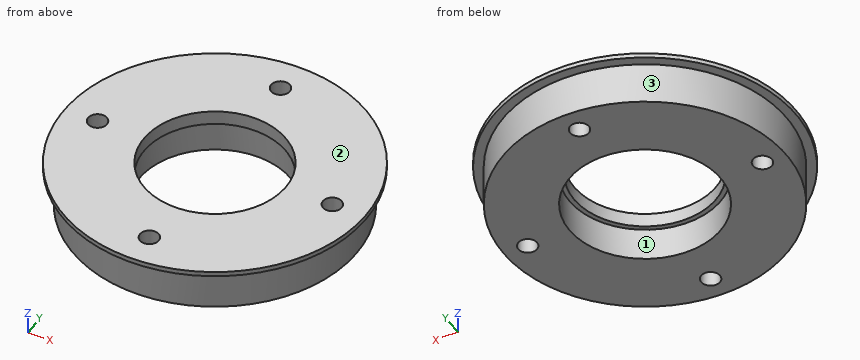
```python
from build123d import *

# Parameters (mm, degrees)
SKETCH1_R           = 29.9974
SKETCH1_R_2         = 16
BOSS_EXTRUDE1_DEPTH = 7
SKETCH2_R           = 2
CUT_EXTRUDE1_DEPTH  = 10
SKETCH3_R           = 16
SKETCH3_R_2         = 15
BOSS_EXTRUDE2_DEPTH = 1
BOSS_EXTRUDE3_START = 3
SKETCH1_3_R         = 29.9974
SKETCH1_3_R_2       = 16
BOSS_EXTRUDE3_DEPTH = 3
BOSS_EXTRUDE4_START = 2
SKETCH3_2_R         = 16
SKETCH3_2_R_2       = 15
BOSS_EXTRUDE4_DEPTH = 2
SKETCH4_R           = 31.9974
SKETCH4_R_2         = 29.9974
BOSS_EXTRUDE5_DEPTH = 1
CUT_EXTRUDE3_START  = -1
SKETCH5_R           = 16
SKETCH5_R_2         = 15
CUT_EXTRUDE3_DEPTH  = 1
SKETCH6_R           = 3
SKETCH6_R_2         = 2
BOSS_EXTRUDE6_DEPTH = 3
CHAMFER1_SIZE       = 3
CUT_EXTRUDE4_START  = -10
SKETCH7_R           = 2
CUT_EXTRUDE4_DEPTH  = 10
BOSS_EXTRUDE7_START = 1
SKETCH8_R           = 16
SKETCH8_R_2         = 15
BOSS_EXTRUDE7_DEPTH = 1


# Read off the part's stored shape, not the designer's step: Cut-Extrude5
with BuildPart() as part:
    # Sketch1 → Boss-Extrude1 (new body)
    with BuildSketch(Plane.XY):
        Circle(SKETCH1_R)
        Circle(SKETCH1_R_2, mode=Mode.SUBTRACT)
    extrude(amount=-BOSS_EXTRUDE1_DEPTH)

    # Sketch2 → Cut-Extrude1 (cut)
    with BuildSketch(Plane.XY):
        with Locations((25, 0)):
            Circle(SKETCH2_R)
        with Locations((0, -25)):
            Circle(SKETCH2_R)
        with Locations((-25, 0)):
            Circle(SKETCH2_R)
        with Locations((0, 25)):
            Circle(SKETCH2_R)
    extrude(amount=-CUT_EXTRUDE1_DEPTH, mode=Mode.SUBTRACT)

    # Sketch3 → Boss-Extrude2 (add)
    with BuildSketch(Plane.XY):
        Circle(SKETCH3_R)
        Circle(SKETCH3_R_2, mode=Mode.SUBTRACT)
    extrude(amount=-BOSS_EXTRUDE2_DEPTH)

    # Sketch1<3> → Boss-Extrude3 (add)
    with BuildSketch(Plane.XY.offset(BOSS_EXTRUDE3_START)):
        Circle(SKETCH1_3_R)
        Circle(SKETCH1_3_R_2, mode=Mode.SUBTRACT)
    extrude(amount=-BOSS_EXTRUDE3_DEPTH)

    # Sketch3<2> → Boss-Extrude4 (add)
    with BuildSketch(Plane.XY.offset(BOSS_EXTRUDE4_START)):
        Circle(SKETCH3_2_R)
        Circle(SKETCH3_2_R_2, mode=Mode.SUBTRACT)
    extrude(amount=-BOSS_EXTRUDE4_DEPTH)

    # Sketch4 → Boss-Extrude5 (add)
    with BuildSketch(Plane.XY.offset(3)):
        Circle(SKETCH4_R)
        Circle(SKETCH4_R_2, mode=Mode.SUBTRACT)
    extrude(amount=-BOSS_EXTRUDE5_DEPTH)

    # Sketch5 → Cut-Extrude3 (cut)
    with BuildSketch(Plane(origin=(0, 0, -1), x_dir=(-1, 0, 0), z_dir=(0, 0, -1)).offset(CUT_EXTRUDE3_START)):
        with Locations(Location((0, 0, 0), (0, 0, 180))):
            Circle(SKETCH5_R)
        with Locations(Location((0, 0, 0), (0, 0, 180))):
            Circle(SKETCH5_R_2, mode=Mode.SUBTRACT)
    extrude(amount=CUT_EXTRUDE3_DEPTH, mode=Mode.SUBTRACT)

    # Sketch6 → Boss-Extrude6 (add)
    # profile 1 of 4: a face of its own
    with BuildSketch(Plane(origin=(0, 0, -7), x_dir=(-1, 0, 0), z_dir=(0, 0, -1))):
        with Locations(Location((-25, 0, 0), (0, 0, 180))):
            Circle(SKETCH6_R)
        with Locations(Location((-25, 0, 0), (0, 0, 180))):
            Circle(SKETCH6_R_2, mode=Mode.SUBTRACT)
    # profile 2 of 4: a face of its own
    with BuildSketch(Plane(origin=(0, 0, -7), x_dir=(-1, 0, 0), z_dir=(0, 0, -1))):
        with Locations(Location((0, -25, 0), (0, 0, 180))):
            Circle(SKETCH6_R)
        with Locations(Location((0, -25, 0), (0, 0, 180))):
            Circle(SKETCH6_R_2, mode=Mode.SUBTRACT)
    # profile 3 of 4: a face of its own
    with BuildSketch(Plane(origin=(0, 0, -7), x_dir=(-1, 0, 0), z_dir=(0, 0, -1))):
        with Locations(Location((25, 0, 0), (0, 0, 180))):
            Circle(SKETCH6_R)
        with Locations(Location((25, 0, 0), (0, 0, 180))):
            Circle(SKETCH6_R_2, mode=Mode.SUBTRACT)
    # profile 4 of 4: a face of its own
    with BuildSketch(Plane(origin=(0, 0, -7), x_dir=(-1, 0, 0), z_dir=(0, 0, -1))):
        with Locations(Location((0, 25, 0), (0, 0, 180))):
            Circle(SKETCH6_R)
        with Locations(Location((0, 25, 0), (0, 0, 180))):
            Circle(SKETCH6_R_2, mode=Mode.SUBTRACT)
    extrude(amount=BOSS_EXTRUDE6_DEPTH)

    # Chamfer1
    # the kernel refuses this chamfer: 3 mm, written as the material it adds along each edge
    with BuildSketch(Plane(origin=(25, 0, -7), x_dir=(1, 0, 0), z_dir=(0, 1, 0))) as chamfer1_piece_1_section:
        Polygon((3 + CHAMFER1_SIZE, 0), (3, CHAMFER1_SIZE), (3, 0), align=None)
    chamfer1_piece_1 = revolve(axis=Axis((25, 0, -7), (0, 0, -1)), mode=Mode.PRIVATE)
    chamfer1_piece_1 = chamfer1_piece_1 & Plane(origin=(0, 0, -8.42256149), x_dir=(1, 0, 0), z_dir=(0, 0, 1)) * Cylinder(29.9974, 25, mode=Mode.PRIVATE)
    chamfer1_piece_1 = split(chamfer1_piece_1, bisect_by=Plane(origin=(20.492585696, 0, -10), z_dir=(0, 0, 1)), keep=Keep.TOP, mode=Mode.PRIVATE)
    add(chamfer1_piece_1)
    with BuildSketch(Plane(origin=(0, -25, -7), x_dir=(1, 0, 0), z_dir=(0, 1, 0))) as chamfer1_piece_2_section:
        Polygon((3 + CHAMFER1_SIZE, 0), (3, CHAMFER1_SIZE), (3, 0), align=None)
    chamfer1_piece_2 = revolve(axis=Axis((0, -25, -7), (0, 0, -1)), mode=Mode.PRIVATE)
    chamfer1_piece_2 = chamfer1_piece_2 & Plane(origin=(0, 0, -8.422561428), x_dir=(1, 0, 0), z_dir=(0, 0, 1)) * Cylinder(29.9974, 25, mode=Mode.PRIVATE)
    chamfer1_piece_2 = split(chamfer1_piece_2, bisect_by=Plane(origin=(-4.507414242, -25, -10), z_dir=(0, 0, 1)), keep=Keep.TOP, mode=Mode.PRIVATE)
    add(chamfer1_piece_2)
    with BuildSketch(Plane(origin=(-25, 0, -7), x_dir=(1, 0, 0), z_dir=(0, 1, 0))) as chamfer1_piece_3_section:
        Polygon((3 + CHAMFER1_SIZE, 0), (3, CHAMFER1_SIZE), (3, 0), align=None)
    chamfer1_piece_3 = revolve(axis=Axis((-25, 0, -7), (0, 0, -1)), mode=Mode.PRIVATE)
    chamfer1_piece_3 = chamfer1_piece_3 & Plane(origin=(0, 0, -8.422561427), x_dir=(1, 0, 0), z_dir=(0, 0, 1)) * Cylinder(29.9974, 25, mode=Mode.PRIVATE)
    chamfer1_piece_3 = split(chamfer1_piece_3, bisect_by=Plane(origin=(-29.507414241, 0, -10), z_dir=(0, 0, 1)), keep=Keep.TOP, mode=Mode.PRIVATE)
    add(chamfer1_piece_3)
    with BuildSketch(Plane(origin=(0, 25, -7), x_dir=(1, 0, 0), z_dir=(0, 1, 0))) as chamfer1_piece_4_section:
        Polygon((3 + CHAMFER1_SIZE, 0), (3, CHAMFER1_SIZE), (3, 0), align=None)
    chamfer1_piece_4 = revolve(axis=Axis((0, 25, -7), (0, 0, -1)), mode=Mode.PRIVATE)
    chamfer1_piece_4 = chamfer1_piece_4 & Plane(origin=(0, 0, -8.422561436), x_dir=(1, 0, 0), z_dir=(0, 0, 1)) * Cylinder(29.9974, 25, mode=Mode.PRIVATE)
    chamfer1_piece_4 = split(chamfer1_piece_4, bisect_by=Plane(origin=(-4.50741425, 25, -10), z_dir=(0, 0, 1)), keep=Keep.TOP, mode=Mode.PRIVATE)
    add(chamfer1_piece_4)

    # Sketch7 → Cut-Extrude4 (cut)
    with BuildSketch(Plane(origin=(0, 0, 0), x_dir=(-1, 0, 0), z_dir=(0, 0, -1)).offset(CUT_EXTRUDE4_START)):
        with Locations(Location((-25, 0, 0), (0, 0, 180))):
            Circle(SKETCH7_R)
        with Locations(Location((0, 25, 0), (0, 0, 180))):
            Circle(SKETCH7_R)
        with Locations(Location((25, 0, 0), (0, 0, 180))):
            Circle(SKETCH7_R)
        with Locations(Location((0, -25, 0), (0, 0, 180))):
            Circle(SKETCH7_R)
    extrude(amount=CUT_EXTRUDE4_DEPTH, mode=Mode.SUBTRACT)

    # Sketch8 → Boss-Extrude7 (add)
    with BuildSketch(Plane.XY.offset(2).offset(BOSS_EXTRUDE7_START)):
        Circle(SKETCH8_R)
        Circle(SKETCH8_R_2, mode=Mode.SUBTRACT)
    extrude(amount=-BOSS_EXTRUDE7_DEPTH)

    # Cut-Extrude5 outline → Cut-Extrude5 (revolve, cut)
    with BuildSketch(Plane(origin=(25, 0, 0), x_dir=(1, 0, 0), z_dir=(0, -1, 0))):
        Polygon((2, -7), (2, -10), (3, -10), (6, -7), align=None)
    revolve(axis=Axis((25, 0, 0), (0, 0, 1)), mode=Mode.SUBTRACT)

    # Cut-Extrude5 2 outline → Cut-Extrude5 2 (revolve, cut)
    with BuildSketch(Plane.XZ.offset(25)):
        Polygon((2, -7), (2, -10), (3, -10), (6, -7), align=None)
    revolve(axis=Axis((0, -25, 0), (0, 0, 1)), mode=Mode.SUBTRACT)

    # Cut-Extrude5 3 outline → Cut-Extrude5 3 (revolve, cut)
    with BuildSketch(Plane(origin=(-25, 0, 0), x_dir=(1, 0, 0), z_dir=(0, -1, 0))):
        Polygon((2, -7), (2, -10), (3, -10), (6, -7), align=None)
    revolve(axis=Axis((-25, 0, 0), (0, 0, 1)), mode=Mode.SUBTRACT)

    # Cut-Extrude5 4 outline → Cut-Extrude5 4 (revolve, cut)
    with BuildSketch(Plane.XZ.offset(-25)):
        Polygon((2, -7), (2, -10), (3, -10), (6, -7), align=None)
    revolve(axis=Axis((0, 25, 0), (0, 0, 1)), mode=Mode.SUBTRACT)


solid = part.part
```
CAD build for the part. Positions are in the model's coordinates, mm. Face numbers are marked on the shaded views. Coordinates: 2 decimals unless noted, no trailing zeros. Write each loop counter-clockwise with the first axis right and the second up, starting at its lowest first coordinate (ties: lowest second). Pieces come first, ordered by that corner, then holes. Notation, with made-up numbers: (76.5, -38) -> (135.5, -38) arc R23 cw to (135.5, -6) -> close; hole circle Ø7 at (75.25, -24). An arc over 180 degrees is marked (long way). Return JSON: item names as keys, results as strings. Group by question number.
Q1. Drill centre lines: line 1 (Y direction, x = 0, z = 1.5); line 2 (Y direction, x = 0, z = -4); line 3 (Y direction, x = 25, z = 0). Where is each one in solid material? Low to high.
Q2. Cut at A-A, the plane x = 0. Give the cut face in (y, z), then the cut area to 3 significant figures.
Q3. Flat gauge pins, fed straight in: pin 1 (3.5 mm diameter, centred on x = 0, y = -25, fed in from -Z); pin 2 (5 mm diameter, centred on x = 19.5, z = -1, fed in from +Y); pin 3 (4 mm diameter, centred on y = 2.5, z = -1.5, fed in from -X); pin 4 (4 mm diameter, centred on x = -3, z = -1, fed in from -Y). Where does each tip first touch, or does it go through?
Q4. Cut at C-C, the plane z = -1.75. Give the cut face in (x, y), then the cut area to 3 significant figures.
Q5. Cut at D-D, the plane x = -25. Give the cut face in (y, z).
Q6. Pull direction X, two halves, no side cores. Call the marked faces 1, 2 and 3: released by +X, released by -X, zero draft, split by the parting line, or undercut.
Returned:
{
 "1": {"line 1": "y = -30 to -27, -23 to -15, 15 to 23, 27 to 30", "line 2": "y = -30 to -27, -23 to -16, 16 to 23, 27 to 30", "line 3": "y = -16.58 to -2, 2 to 16.58"},
 "2": {"outline": "(-32, 2) -> (-30, 2) -> (-30, -7) -> (-27, -7) -> (-27, 3) -> (-32, 3) -> close; (-23, -7) -> (-16, -7) -> (-16, 0) -> (-15, 0) -> (-15, 3) -> (-23, 3) -> close; (15, 0) -> (16, 0) -> (16, -7) -> (23, -7) -> (23, 3) -> (15, 3) -> close; (27, -7) -> (30, -7) -> (30, 2) -> (32, 2) -> (32, 3) -> (27, 3) -> close", "area": "210 mm2"},
 "3": {"pin 1": "passes through", "pin 2": "stops at y = 24.72", "pin 3": "stops at x = -29.99", "pin 4": "stops at y = -29.98"},
 "4": {"outline": "circle Ø59.99 at (0, 0); hole circle Ø4 at (-25, 0); hole circle Ø32 at (0, 0); hole circle Ø4 at (0, -25); hole circle Ø4 at (0, 25); hole circle Ø4 at (25, 0)", "area": "1,970 mm2"},
 "5": {"outline": "(-19.97, 2) -> (-16.58, 2) -> (-16.58, -7) -> (-2, -7) -> (-2, 3) -> (-19.97, 3) -> close; (2, -7) -> (16.58, -7) -> (16.58, 2) -> (19.97, 2) -> (19.97, 3) -> (2, 3) -> close"},
 "6": {"face 1": "undercut", "face 2": "zero draft", "face 3": "split by the parting line"}
}
